For this review, take the finished solid that the model builds, in its own axes (mm). A direction names the side the tool comes from. Coordinates: 2 decimals unless noted, no trailing zeros. Loops run counter-clockwise (first coordinate to the right, second up) from the corner with the lowest first, then second, coordinate; pieces in that order, holes last. Notation, with made-up numbers: M 61.25,88 L 110.25,88 A11 cw 110.25,106 Z; hole C -22,-1 d2. An arc over 180 degrees is marked long. Answer as a JSON object with one key per item and string values. Group by question number.
Item 1: Insertion check: pin 1 (9 mm diameter, centred on x = 50.5, z = 6.5, fed in from +Y). The pin has a flat end and moves straight along its axis. Give the tip position at first contact, or say it passes through.
Item 2: Add section B-B (x = 61.5). State the section outline as (y, z) points.
Item 3: Tool access review of faces 1 (the face through (5.715, -22, 0)), 2 (the face through (13.093, -29.381, -0.11)), 3 (the face through (37, -8, 7)): name each direction out of +Z, -Z, +X, -X, +Y, -Y from which nothing blocks a thin tool from reaching the whole face with its end or side.
Item 4: Mouldability with a two-part tool opening along Z and no side actions: class faces 4 (the face through (36, -23, 12.5)), 5 (the face through (55.093, -29.381, -0.11)), 6 (the face through (36, -38, 0)) as +Z half, -Z half, draft (parallel to the pull), parting line (faces both ways), or undercut.
Item 5: Add section C-C (z = 5.5). State the section outline as (x, y) points, then the cut area to 3 significant figures.
Item 6: Wall thickness on L1, parallel to Y at x = 55.5, z = 9.75; L2, parallel to Z at x = 59, y = -35.5; L3, parallel to Z at x = 11.5, y = -7: over which ranges is each line inside the solid? List them lowest first. Write a range as from..to.
Item 7: Add section A-A (y = -33.5). State the section outline as (x, z) points.
from build123d import *

# Parameters (mm, degrees)
SKETCH1_W             = 61.75
SKETCH1_H             = 38
BOSS_EXTRUDE1_DEPTH   = 12.5
CUT_EXTRUDE1_REACH    = 75.575
M6_TAPPED_HOLE1_D     = 5
M6_TAPPED_HOLE1_DEPTH = 17
M6_TAPPED_HOLE1_TIP   = 1.502151548


with BuildPart() as part:
    # Sketch1 → Boss-Extrude1 (new, symmetric)
    with BuildSketch(Plane.XY):
        with Locations((36.590437788, -19)):
            Rectangle(SKETCH1_W, SKETCH1_H)
    extrude(amount=BOSS_EXTRUDE1_DEPTH, both=True)

    # Sketch2 → Cut-Extrude1 (cut, up to next)
    with BuildSketch(Plane(origin=(67.465437788, 0, 0), x_dir=(0, 0, -1), z_dir=(1, 0, 0)), mode=Mode.PRIVATE) as cut_extrude1_sk1:
        with BuildLine():
            Line((1.964101615, -6), (12.5, -6))
            Line((12.5, -6), (12.5, 0))
            Line((12.5, 0), (-12.5, 0))
            Line((-12.5, 0), (-12.5, -8))
            Line((-12.5, -8), (-1.5, -8))
            ThreePointArc((-1.5, -8), (0.5, -7.464101615), (1.964101615, -6))
        make_face()
    cut_extrude1_tool1 = extrude(cut_extrude1_sk1.sketch, amount=-CUT_EXTRUDE1_REACH, mode=Mode.PRIVATE) & part.part
    add(cut_extrude1_tool1.solids().sort_by_distance((67.465438, -3.603515, 0.874459))[0], mode=Mode.SUBTRACT)

    # M6 Tapped Hole1
    with Locations(Plane(origin=(0, -38, 0), x_dir=(-1, 0, 0), z_dir=(0, -1, 0))):
        with Locations((-15.590437788, 0), (-57.590437788, 0)):
            Hole(M6_TAPPED_HOLE1_D / 2, depth=M6_TAPPED_HOLE1_DEPTH)
            with Locations((0, 0, -(M6_TAPPED_HOLE1_DEPTH + M6_TAPPED_HOLE1_TIP / 2))):  # 118° drill point
                Cone(0, M6_TAPPED_HOLE1_D / 2, M6_TAPPED_HOLE1_TIP, mode=Mode.SUBTRACT)


solid = part.part
From the geometry:
{
 "1": {"pin 1": "stops at y = -8"},
 "2": {"outline": "M -38,-12.5 L -6,-12.5 L -6,-1.96 A4 cw -8,1.5 L -8,12.5 L -38,12.5 Z"},
 "3": {"face 1": "+Z, -Z, -X, +Y, -Y", "face 2": "-Y", "face 3": "+Z, +X, -X, +Y"},
 "4": {"face 4": "+Z half", "face 5": "undercut", "face 6": "draft"},
 "5": {"outline": "M 5.72,-38 L 67.47,-38 L 67.47,-8 L 5.72,-8 Z", "area": "1,850 mm²"},
 "6": {"L1": "y = -38..-8", "L2": "z = -12.5..-2.06, 2.06..12.5", "L3": "z = -12.5..-1.15"},
 "7": {"outline": "M 5.72,-12.5 L 67.47,-12.5 L 67.47,12.5 L 5.72,12.5 Z; hole C 15.59,0 d5; hole C 57.59,0 d5"}
}
